```python
from build123d import *

# Parameters (mm, degrees)
SALIENTE_EXTRUIR1_DEPTH                         = 5
CROQUIS6_R                                      = 1.6
CORTAR_EXTRUIR4_DEPTH                           = 10
CROQUIS8_R                                      = 10.5
CORTAR_EXTRUIR5_DEPTH                           = 4
CROQUIS9_R                                      = 9.5
CORTAR_EXTRUIR6_DEPTH                           = 4
CSK_FOR_M3_FLAT_HEAD_MACHINE_SCREW1_D           = 3.4
CSK_FOR_M3_FLAT_HEAD_MACHINE_SCREW1_CSINK_D     = 6.3
CSK_FOR_M3_FLAT_HEAD_MACHINE_SCREW1_CSINK_ANGLE = 90


with BuildPart() as part:
    # Croquis1 → Saliente-Extruir1 (new body)
    with BuildSketch(Plane(origin=(0, 0, 0), x_dir=(1, 0, 0), z_dir=(0, 1, 0))):
        with BuildLine():
            Line((-9.944316368, 11.229896347), (-9.944316368, 72.824175738))
            ThreePointArc((-9.944316368, 72.824175738), (0.028101663, 73.499994628), (10, 72.816550317))
            Line((10, 72.816550317), (10, 11.180339887))
            ThreePointArc((10, 11.180339887), (13.008976456, 7.467699215), (14.697533703, 2.997082424))
            Line((14.697533703, 2.997082424), (68.039744383, -27.800057271))
            ThreePointArc((68.039744383, -27.800057271), (63.468798846, -37.066987644), (57.643462165, -45.601329691))
            Line((57.643462165, -45.601329691), (4.689417529, -14.24813543))
            ThreePointArc((4.689417529, -14.24813543), (-0.033608107, -14.99996235), (-4.753217335, -14.226978772))
            Line((-4.753217335, -14.226978772), (-58.095428015, -45.024118467))
            ThreePointArc((-58.095428015, -45.024118467), (-63.835352365, -36.432098327), (-68.313641042, -27.120037751))
            Line((-68.313641042, -27.120037751), (-14.68380565, 3.06363373))
            ThreePointArc((-14.68380565, 3.06363373), (-12.973359619, 7.529405035), (-9.944316368, 11.229896347))
        make_face()
    extrude(amount=SALIENTE_EXTRUIR1_DEPTH)

    # Croquis6 → Cortar-Extruir4 (cut, symmetric)
    with BuildSketch(Plane(origin=(0, 5, 0), x_dir=(1, 0, 0), z_dir=(0, 1, 0))):
        with Locations(Location((0, 69, 0), (0, 0, 270))):
            Circle(CROQUIS6_R)
        with Locations(Location((59.755752861, -34.5, 0), (0, 0, 270))):
            Circle(CROQUIS6_R)
        with Locations(Location((-59.755752861, -34.5, 0), (0, 0, 270))):
            Circle(CROQUIS6_R)
    extrude(amount=CORTAR_EXTRUIR4_DEPTH, both=True, mode=Mode.SUBTRACT)

    # Croquis8 → Cortar-Extruir5 (cut)
    with BuildSketch(Plane.XZ):
        with Locations(Location((0, 0, 0), (0, 0, 270))):
            Circle(CROQUIS8_R)
    extrude(amount=-CORTAR_EXTRUIR5_DEPTH, mode=Mode.SUBTRACT)

    # Croquis9 → Cortar-Extruir6 (cut)
    with BuildSketch(Plane(origin=(0, 5, 0), x_dir=(1, 0, 0), z_dir=(0, 1, 0))):
        with Locations(Location((0, 0, 0), (0, 0, 270))):
            Circle(CROQUIS9_R)
    extrude(amount=-CORTAR_EXTRUIR6_DEPTH, mode=Mode.SUBTRACT)

    # CSK for M3 Flat Head Machine Screw1 (through all)
    with Locations(Plane(origin=(0, 5, 0), x_dir=(1, 0, 0), z_dir=(0, 1, 0))):
        with Locations((-59.755752861, -34.5), (0, 69), (59.755752861, -34.5)):
            CounterSinkHole(CSK_FOR_M3_FLAT_HEAD_MACHINE_SCREW1_D / 2, CSK_FOR_M3_FLAT_HEAD_MACHINE_SCREW1_CSINK_D / 2, counter_sink_angle=CSK_FOR_M3_FLAT_HEAD_MACHINE_SCREW1_CSINK_ANGLE)


solid = part.part
```
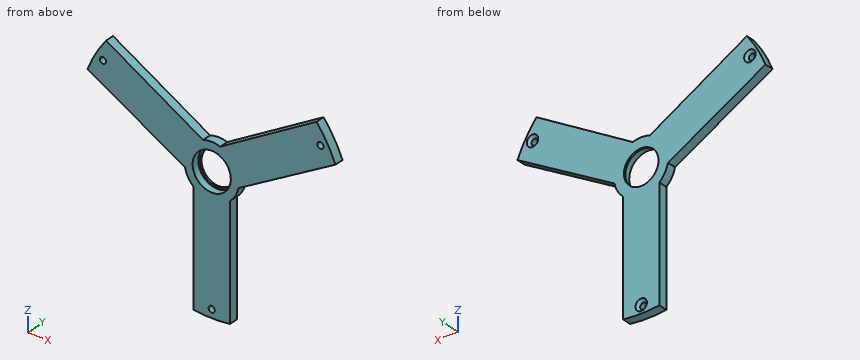
For this review, take the finished solid that the model builds, in its own axes (mm). Round coordinates to 2 decimals unless told otherwise and drop trailing zeros. Write each loop counter-clockwise with the first axis right and the second up, starting at its lowest first coordinate (ties: lowest second). Pieces come first, ordered by that corner, then holes. Notation, with made-up numbers: (36.25, -29.75) - (79.25, -29.75) arc R20 ccw to (79.25, -23.75) - close; hole circle Ø2 at (-5.5, -39). An arc over 180 degrees is marked (long way). Answer as CSV lines item,"result". Start each with the question number.
(1) Add section C-C, the plane y = 1.15. State the section outline as (x, z) points.
(2) For line 1 (X direction, y = 2.7, z = 34.5); line 2 (X direction, y = 3.3, z = -62); line 3 (Z direction, x = -59, y = 2.4), list the stretches that pass through material, from the lowest coordinate up.
(3) Add section B-B, the plane x = 0. State the section outline as (y, z) points.
(4) Add section A-A, the plane z = -69. State the section outline as (x, y) points, plus the area to 3 significant figures.
(5) Add section D-D, the plane z = 34.5. State the section outline as (x, y) points, plus the area to 3 significant figures.
(6) For pin 1 (1.5 mm diameter, centred on y = 2.5, z = -35, fed in from -X); pin 2 (4 mm diameter, centred on x = 59.76, z = 34.5, fed in from +Y); pin 3 (1.5 mm diameter, centred on y = 3, z = -45, fed in from +X); pin 4 (23 mm diameter, centred on x = -4, z = 3.5, fed in from -Y), all flat-tipped, find the tip position at first contact; note any pin that passes through.
From the geometry:
1,outline,"(-68.31, 27.12) - (-14.68, -3.06) arc R15 ccw to (-9.94, -11.23) - (-9.94, -72.82) arc R73.5 ccw to (10, -72.82) - (10, -11.18) arc R15 ccw to (14.7, -3) - (68.04, 27.8) arc R73.5 ccw to (57.64, 45.6) - (4.69, 14.25) arc R15 ccw to (-4.75, 14.23) - (-58.1, 45.02) arc R73.5 ccw to start; hole circle Ø3.4 at (-59.76, 34.5); hole circle Ø21 at (0, 0); hole circle Ø3.4 at (0, -69); hole circle Ø3.4 at (59.76, 34.5)"
2,line 1,"x = -64.9 to -61.46, -58.06 to -39.87, 38.89 to 58.06, 61.46 to 64.9"
2,line 2,"x = -9.94 to 10"
2,line 3,"z = 21.88 to 32.98, 36.02 to 43.83"
3,outline,"(0, -73.5) - (5, -73.5) - (5, -72.15) - (3.55, -70.7) - (0, -70.7) - close; (0, -67.3) - (3.55, -67.3) - (5, -65.85) - (5, -9.5) - (4, -9.5) - (4, -10.5) - (0, -10.5) - close; (0, 10.5) - (4, 10.5) - (4, 9.5) - (5, 9.5) - (5, 15) - (0, 15) - close"
4,outline,"(-9.94, 0) - (-1.7, 0) - (-1.7, 3.55) - (-3.15, 5) - (-9.94, 5) - close; (1.7, 0) - (10, 0) - (10, 5) - (3.15, 5) - (1.7, 3.55) - close"
4,area,"80.6 mm²"
5,outline,"(-64.9, 0) - (-61.46, 0) - (-61.46, 3.55) - (-62.91, 5) - (-64.9, 5) - close; (-58.06, 0) - (-39.87, 0) - (-39.87, 5) - (-56.61, 5) - (-58.06, 3.55) - close; (38.89, 0) - (58.06, 0) - (58.06, 3.55) - (56.61, 5) - (38.89, 5) - close; (61.46, 0) - (64.9, 0) - (64.9, 5) - (62.91, 5) - (61.46, 3.55) - close"
5,area,"217 mm²"
6,pin 1,"stops at x = -9.94"
6,pin 2,"stops at y = 3.85"
6,pin 3,"stops at x = 10"
6,pin 4,"stops at y = 0"
